Source: three-view drawing plus pictorial views. Frame: mm from the lowest corner of the part. A direction names the side the tool comes from. Give positions to 0.01 mm unless a question says otherwise; leave off trailing zeros. Write each loop counter-clockwise with the first axis right and the second up, starting at its lowest first coordinate (ties: lowest second). Pieces come first, ordered by that corner, then holes. Notation, with made-up numbers: M 8.5,79 L 56.5,79 A23 cw 56.5,114 Z; hole C 89.5,25.5 d2. An arc over 180 degrees is marked long. Return JSON: item names as keys, results as strings.
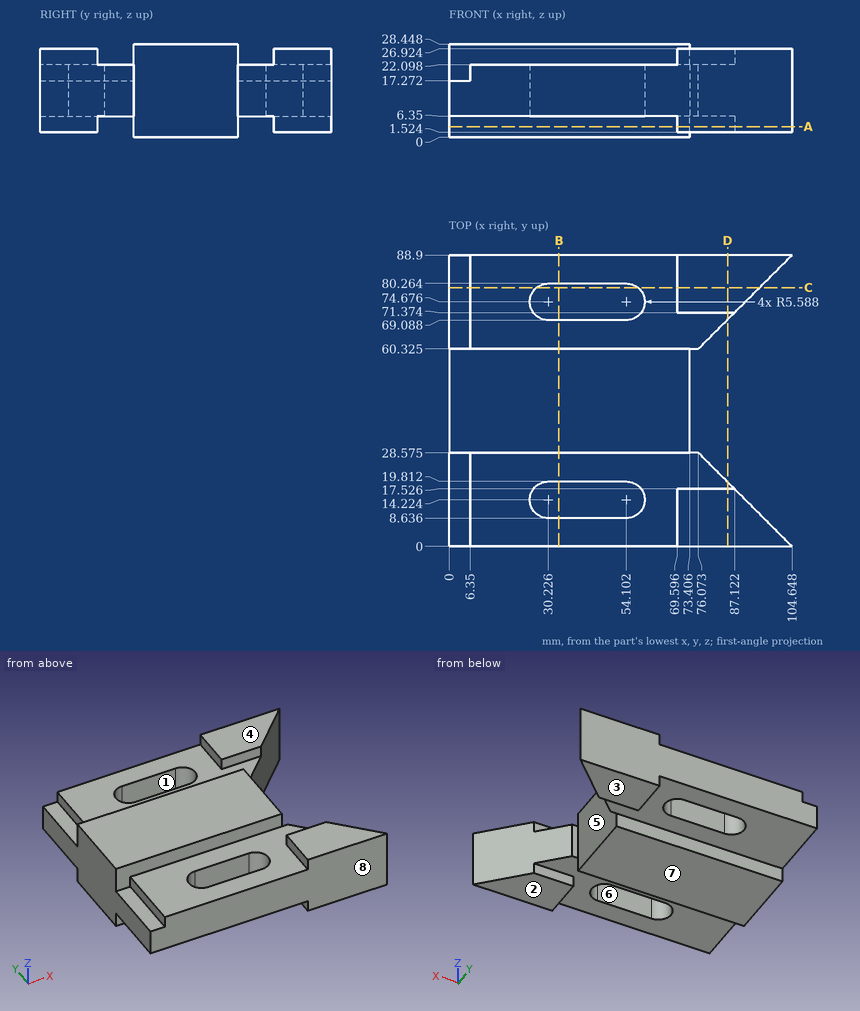
1) Contact query for flat-ended pins moving along their axis: pin 1 Ø5 at (y, z) = (15.5, 20) entering from -X; pin 2 Ø2 at (y, z) = (36, 18.5) entering from +X; pin 3 Ø1.9 at (x, y) = (2.5, 79) entering from +Z; pin 4 Ø1.4 at (x, z) = (75.5, 24.5) entering from -Y. Output: stop coordinate, or through.
Numbers:
{"pin 1": "stops at x = 6.35", "pin 2": "stops at x = 73.41", "pin 3": "stops at z = 17.27", "pin 4": "stops at y = 0"}
2) Cut plane D-D, the plane x = 85. Return the cut outline in (y, z).
Numbers:
{"outline": "M 0,1.52 L 17.53,1.52 L 17.53,6.35 L 19.65,6.35 L 19.65,22.1 L 17.53,22.1 L 17.53,26.92 L 0,26.92 Z; M 69.25,6.35 L 71.37,6.35 L 71.37,1.52 L 88.9,1.52 L 88.9,26.92 L 71.37,26.92 L 71.37,22.1 L 69.25,22.1 Z"}
3) Cut plane C-C, the plane y = 79. Return the cut outline in (x, z).
Numbers:
{"outline": "M 0,6.35 L 26.69,6.35 L 26.69,22.1 L 6.35,22.1 L 6.35,17.27 L 0,17.27 Z; M 57.64,6.35 L 69.6,6.35 L 69.6,1.52 L 94.75,1.52 L 94.75,26.92 L 69.6,26.92 L 69.6,22.1 L 57.64,22.1 Z"}
4) Line query: line 1 (Y direction, x = 38, z = 21); line 2 (Y direction, x = 73.5, z = 10) (3 decimals); line 3 (Z direction, x = 82, y = 13). Output: solid intervals per line, ascending. Write a range as [from, to].
Numbers:
{"line 1": "y = [0, 8.64], [19.81, 69.09], [80.26, 88.9]", "line 2": "y = [0, 28.575], [60.325, 88.9]", "line 3": "z = [1.52, 26.92]"}
5) Draft query along Y for the marked faces 6, 7 and 8. Return one class per face: released by +Y, released by -Y, zero draft, split by the parting line, or undercut.
Numbers:
{"face 6": "undercut", "face 7": "zero draft", "face 8": "released by -Y"}
6) Cut plane A-A, the plane z = 3.25. Return the cut outline in (x, y) (3 decimals), then the cut area to 3 significant figures.
Numbers:
{"outline": "M 0,28.575 L 73.406,28.575 L 73.406,60.325 L 0,60.325 Z; M 69.596,0 L 104.648,0 L 87.122,17.526 L 69.596,17.526 Z; M 69.596,71.374 L 87.122,71.374 L 104.648,88.9 L 69.596,88.9 Z", "area": "3,250 mm²"}
7) Set-up query: the marked faces 1, 2, 3, 4 and 5. Return all of +Z, -Z, +X, -X, +Y, -Y with unobstructed straight access to the full face (end or side cutting, diameter ignored); none if empty.
Numbers:
{"face 1": "+Z, -Z", "face 2": "-Z, +X, -X, -Y", "face 3": "-Z, +X, -X, +Y", "face 4": "+Z, +X, -X, +Y", "face 5": "+Z, -Z, +X"}
8) Cut plane B-B, the plane x = 33.5. Return the cut outline in (y, z) (3 decimals).
Numbers:
{"outline": "M 0,6.35 L 8.636,6.35 L 8.636,22.098 L 0,22.098 Z; M 19.812,6.35 L 28.575,6.35 L 28.575,0 L 60.325,0 L 60.325,6.35 L 69.088,6.35 L 69.088,22.098 L 60.325,22.098 L 60.325,28.448 L 28.575,28.448 L 28.575,22.098 L 19.812,22.098 Z; M 80.264,6.35 L 88.9,6.35 L 88.9,22.098 L 80.264,22.098 Z"}
